Autodesk Inventor part; units mm, degrees
ref_plane "IP1_XY" through (0, 0, 0) normal (1, 0, 0) x (0, 0, -1)
ref_plane "IP1_YZ" through (0, 0, 0) normal (0, 0, -1) x (0, 1, 0)
ref_plane "IP1_ZX" through (0, 0, 0) normal (0, 1, 0) x (1, 0, 0)
sketch "Skizze_2" plane through (-3.1, 0, 0) normal (1, 0, 0) x (0, 0, -1)
  arc A0 (-1.6711, 0.3843) -> (-1.6711, -0.3843) centre (-1.58, 0) ccw
  arc A1 (-1.1684, -1.2551) -> (-1.6711, -0.3843) centre (-1.8307, -1.0569) ccw
  arc A2 (-1.1684, -1.2551) -> (-0.5027, -1.6394) centre (-0.79, -1.3683) ccw
  arc A3 (0.5027, -1.6394) -> (-0.5027, -1.6394) centre (0, -2.1139) ccw
  arc A4 (0.5027, -1.6394) -> (1.1684, -1.2551) centre (0.79, -1.3683) ccw
  arc A5 (1.6711, -0.3843) -> (1.1684, -1.2551) centre (1.8307, -1.0569) ccw
  arc A6 (1.6711, -0.3843) -> (1.6711, 0.3843) centre (1.58, 0) ccw
  arc A7 (1.1684, 1.2551) -> (1.6711, 0.3843) centre (1.8307, 1.0569) ccw
  arc A8 (1.1684, 1.2551) -> (0.5027, 1.6394) centre (0.79, 1.3683) ccw
  arc A9 (-0.5027, 1.6394) -> (0.5027, 1.6394) centre (0, 2.1139) ccw
  arc A10 (-0.5027, 1.6394) -> (-1.1684, 1.2551) centre (-0.79, 1.3683) ccw
  arc A11 (-1.6711, 0.3843) -> (-1.1684, 1.2551) centre (-1.8307, 1.0569) ccw
sketch "Skizze_3" plane through (0, 0, 0) normal (0, 0, 1) x (1, 0, 0)
  line L0 (-0.1, 0) -> (-0.2997, 0)
  line L1 (-0.2997, 0) -> (-1.4977, 2.075)
  line L2 (-1.4977, 2.075) -> (-0.1, 2.075)
  line L3 (-0.1, 2.075) -> (-0.1, 0)
  line L4 (-0.1, 0) -> (-0.2997, 0)
sketch "Skizze_5" plane through (0, 0, 0) normal (0, 0, 1) x (1, 0, 0)
  line L0 (25, 0) -> (-3.1, 0)
  line L1 (-3.1, 0) -> (-3.1, 3.2288)
  line L2 (-3.1, 3.2288) -> (0, 3.5)
  line L3 (0, 3.5) -> (0, 1.7853)
  line L4 (0, 1.7853) -> (1.028, 1.7853)
  line L5 (1.028, 1.7853) -> (1.4, 2)
  line L6 (1.4, 2) -> (25, 2)
  line L7 (25, 2) -> (25, 0)
  line L8 (25, 0) -> (-3.1, 0)
revolve "Revolution1" add sketch "Skizze_5" angle 360 about axis through (25, 0, 0) along (1, 0, 0)
thread "Thread1"
sketch "Sketch_1" plane through (0, 0, 0) normal (0, 0, 1) x (1, 0, 0)
  line L0 (0.2, 0) -> (-0.1, 0)
  line L1 (-0.1, 1.6853) -> (0.2, 1.6853)
  line L2 (0.2, 1.6853) -> (0.2, 1.7853)
  arc A0 (0, 1.9852) -> (0.2, 1.7853) centre (0.2, 1.9853) ccw
  line L3 (0, 1.9852) -> (-0.1, 1.9852)
  line L4 (-0.1, 1.9852) -> (-0.1, 1.6853)
revolve "Revolution2" add sketch "Sketch_1" angle 360 about axis through (0.2, 0, 0) along (1, 0, 0)
sketch "Sketch_2" plane through (0, 0, 0) normal (0, 0, 1) x (1, 0, 0)
  line L0 (-1.9597, 0) -> (-3.1, 0)
  line L1 (-3.1, 0) -> (-3.1, 1.975)
  line L2 (-3.1, 1.975) -> (-1.9597, 0)
  line L3 (-1.9597, 0) -> (-3.1, 0)
revolve "Revolution3" cut sketch "Sketch_2" angle 360 about axis through (-1.9597, 0, 0) along (1, 0, 0)
sketch "Sketch_3" plane through (0, 0, 0) normal (0, 0, 1) x (1, 0, 0)
  line L0 (50, 0) -> (-3.1, 0)
  line L1 (-3.6, 8.4) -> (-3.6, 2.9081)
  line L2 (-3.6, 2.9081) -> (-3.1, 2.9081)
  arc A0 (-2.7805, 3.2567) -> (-3.1, 2.9081) centre (-2.75, 2.9081) ccw
  line L3 (-2.7805, 3.2567) -> (-2.7805, 8.4)
  line L4 (-2.7805, 8.4) -> (-3.6, 8.4)
revolve "Revolution4" cut sketch "Sketch_3" angle 360 about axis through (50, 0, 0) along (1, 0, 0)
extrude "Extrusion1" cut sketch "Skizze_2" along normal blind 2.79
revolve "Revolution5" add sketch "Skizze_3" angle 360 about axis through (-0.1, 0, 0) along (1, 0, 0)
ref_plane "IP1_XY" through (0, 0, 0) normal (1, 0, 0) x (0, 0, -1)
ref_plane "IP1_YZ" through (0, 0, 0) normal (0, 0, -1) x (0, 1, 0)
ref_plane "IP1_ZX" through (0, 0, 0) normal (0, 1, 0) x (1, 0, 0)
properties part number "ISO 14580 M4x25"
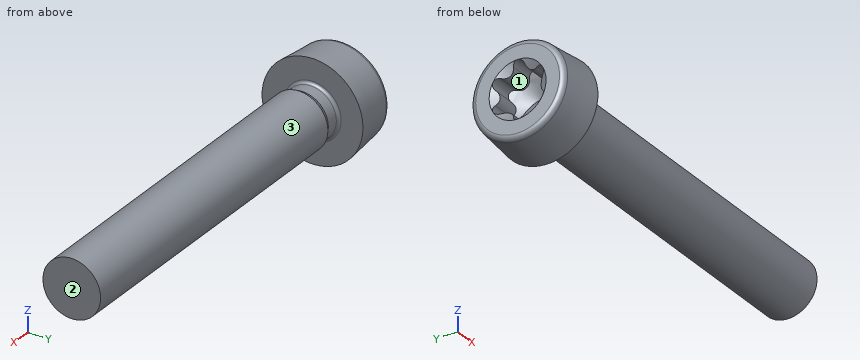
For this review, take the finished solid that the model builds, in its own axes (mm). Face numbers are marked on the shaded views. A direction names the side the tool comes from. Round coordinates to 2 decimals unless told otherwise and drop trailing zeros. Write each loop counter-clockwise with the first axis right and the second up, starting at its lowest first coordinate (ties: lowest second). Pieces come first, ordered by that corner, then holes. Notation, with made-up numbers: M 77.25,-38 L 91.25,-38 A22 ccw 91.25,-14 Z; hole C 64.5,-0.5 d5. An arc over 180 degrees is marked long. One line per item, written item: value. Start each with the question number.
(1) Insertion check: pin 1 (4 mm diameter, centred on x = 10, z = -1, fed in from -Y); pin 2 (1.5 mm diameter, centred on x = 19.5, y = 0.5, fed in from +Z). Each pin has a flat end and moves straight along its axis. Give the tip position at first contact, or say it passes through.
(2) We need section A-A (x = 16). Give the boundary of the cut face in (y, z).
(3) Machinability: for the marked faces 1, 2 and 3, which of the approach directions +Z, -Z, +X, -X, +Y, -Y give a long, thin tool a straight path to every point of the face, cutting with its end or side? Answer none if there is none.
(4) Wall thickness on line 1 (X direction, y = -2.25, z = 1.75); line 2 (Z direction, x = 16.25, y = 0.25): over which ranges is each line inside the solid? List them lowest first.
Result:
1. pin 1: y = -2
1. pin 2: z = 2
2. outline: C 0,0 d4
3. face 1: -X
3. face 2: +Z, -Z, +X, +Y, -Y
3. face 3: +X
4. line 1: -3.1 to 0
4. line 2: -1.98 to 1.98
